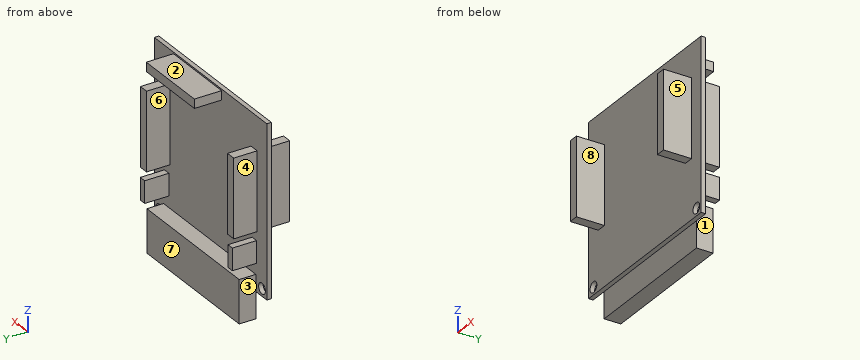
Autodesk Inventor part; units mm, degrees
ref_plane "YZ Plane" through (0, 0, 0) normal (1, 0, 0) x (0, 1, 0)
ref_plane "XZ Plane" through (0, 0, 0) normal (0, 1, 0) x (-1, 0, 0)
ref_plane "XY Plane" through (0, 0, 0) normal (0, 0, 1) x (1, 0, 0)
sketch "Base Board" plane through (0, 0, 0) normal (0, 1, 0) x (-1, 0, 0)
  line L0 (-28.8413, 27.4927) -> (29.6587, 27.4927)
  line L1 (29.6587, 27.4927) -> (29.6587, -28.8073)
  line L2 (29.6587, -28.8073) -> (-28.8413, -28.8073)
  line L3 (-28.8413, -28.8073) -> (-28.8413, 27.4927)
  circle A0 centre (27.1587, -26.3073) radius 1.755
  circle A1 centre (-26.3413, -26.3073) radius 1.755
  line L4 (-23.8413, 16.4927) -> (-20.6413, 16.4927)
  line L5 (-20.6413, 16.4927) -> (-20.6413, -9.3073)
  line L6 (-20.6413, -9.3073) -> (-23.8413, -9.3073)
  line L7 (-23.8413, -9.3073) -> (-23.8413, 16.4927)
  line L8 (24.6587, 16.4927) -> (21.4587, 16.4927)
  line L9 (21.4587, 16.4927) -> (21.4587, -9.3073)
  line L10 (21.4587, -9.3073) -> (24.6587, -9.3073)
  line L11 (24.6587, -9.3073) -> (24.6587, 16.4927)
  point P0 (0, 0)
  dimension "d0" = 58.5
  dimension "d1" = 56.3
  dimension "d2" = 3.51
  dimension "d3" = 2.5
  dimension "d4" = 2.5
  dimension "d5" = 3.51
  dimension "d6" = 2.5
  dimension "d7" = 2.5
  dimension "d19" = 3.2
  dimension "d20" = 25.8
  dimension "d23" = 11
  dimension "d24" = 5
  dimension "d25" = 11
  dimension "d26" = 5
extrude "Base Board Extrusion" add sketch "Base Board" along normal blind 1.5 contours L0 L1 L2 L3 | L4 L5 L6 L7 | L11 L10 L9 L8
sketch "Sketch2" plane through (0, 1.5, 0) normal (0, 1, 0) x (1, 0, 0)
  line L0 (-23.9587, 28.2917) -> (24.0413, 28.2917)
  line L1 (24.0413, 28.2917) -> (24.0413, 23.2917)
  line L2 (24.0413, 23.2917) -> (-23.9587, 23.2917)
  line L3 (-23.9587, 23.2917) -> (-23.9587, 28.2917)
  line L4 (-29.6587, 28.8073) -> (-29.6587, -27.4927)
  point P0 (0, 0)
  dimension "d10" = 48
  dimension "d11" = 5
  dimension "d12" = 5.7
extrude "RightAngleconnectorsBase" add sketch "Sketch2" along normal blind 5.5
sketch "Sketch4" plane through (24.0413, 1.5, -28.2917) normal (0, 0, -1) x (-1, 0, 0)
  line L0 (48, 5.5) -> (0, 5.5)
  line L1 (48, 0) -> (48, 5.5)
  line L2 (0, 5.5) -> (48, 5.5)
  line L3 (48, 5.5) -> (48, 0)
  line L4 (48, 0) -> (0, 0)
  line L5 (0, 0) -> (0, 5.5)
  point P0 (24.0413, -1.5)
extrude "RightAnglePins" add sketch "Sketch4" along normal blind 9.2
extrude "Main IO" add sketch "Base Board" along normal mid plane 18.5 contours L4 L5 L6 L7 | L11 L10 L9 L8
sketch "Sketch6" plane through (0, 1.5, 0) normal (0, 1, 0) x (1, 0, 0)
  line L0 (18.8413, -26.9927) -> (-6.1587, -26.9927)
  line L1 (-6.1587, -26.9927) -> (-6.1587, -23.9927)
  line L2 (-6.1587, -23.9927) -> (18.8413, -23.9927)
  line L3 (18.8413, -23.9927) -> (18.8413, -26.9927)
  line L4 (28.8413, -27.4927) -> (28.8413, 28.8073)
  line L5 (-29.6587, -27.4927) -> (28.8413, -27.4927)
  point P0 (0, 0)
  dimension "d29" = 25
  dimension "d30" = 3
  dimension "d31" = 10
  dimension "d32" = 0.5
extrude "Emulator Pins" add sketch "Sketch6" along normal blind 9
sketch "Sketch7" plane through (0, 1.5, 0) normal (0, 1, 0) x (1, 0, 0)
  line L0 (23.5413, 12.3073) -> (21.2413, 12.3073)
  line L1 (21.2413, 12.3073) -> (21.2413, 19.5573)
  line L2 (21.2413, 19.5573) -> (23.5413, 19.5573)
  line L3 (23.5413, 19.5573) -> (23.5413, 12.3073)
  line L4 (28.8413, -27.4927) -> (28.8413, 28.8073)
  line L5 (23.8413, 9.3073) -> (20.6413, 9.3073)
  line L6 (-29.6587, -27.4927) -> (28.8413, -27.4927)
  line L7 (-24.3587, 12.3073) -> (-22.0587, 12.3073)
  line L8 (-22.0587, 12.3073) -> (-22.0587, 19.5573)
  line L9 (-22.0587, 19.5573) -> (-24.3587, 19.5573)
  line L10 (-24.3587, 19.5573) -> (-24.3587, 12.3073)
  point P0 (0, 0)
  dimension "d35" = 2.3
  dimension "d36" = 7.25
  dimension "d37" = 5.3
  dimension "d38" = 3
extrude "Power Pins" add sketch "Sketch7" along normal blind 8
properties part number "MSP432CoreModule"
Here's how the part is built. I have some questions about the finished solid (model axes, mm). Face numbers are marked on the shaded views. A direction names the side the tool comes from. Round coordinates to 2 decimals unless told otherwise and drop trailing zeros. Write each loop counter-clockwise with the first axis right and the second up, starting at its lowest first coordinate (ties: lowest second). Pieces come first, ordered by that corner, then holes.
Q1. If we section it at D-D on z = 8: Write out the boundary of the cut face in (x, y).
Q2. Will these pins go through, and if not, where does the flat tip stop? P1, Ø5.5, axis at x = 26.34, z = -26.31, coming from the -Y side; P2, Ø6, axis at y = 5, z = 1, coming from the +X side; P3, Ø7, axis at x = 7, z = -34.5, coming from the -Y side.
Q3. If we mould it in two halves opening along X, with no side actions, what happens to the marked faces 5, 6, 7 and 8? For each: +X half, -X half, draft (parallel to the pull), parting line (faces both ways), or undercut.
Q4. If we section it at C-C on x = 0.5: Write out the boundary of the cut face in (y, z).
Q5. If we section it at A-A on y = -6: Write out the boundary of the cut face in (x, z).
Q6. Which directions (+Z, -Z, +X, -X, +Y, -Y) give clear straight access to the entire face, cutting with the end or side of a thin tool? Please do the marked faces 1, 2, 3 and 4.
Q7. If we section it at B-B on y = 4.5: Write out the boundary of the cut face in (x, z), plus the area to 3 significant figures.
Q8. Please list where these lines run through material, in increasing order: probe 1 along X at (y, z) = (2.25, -19); probe 2 along X at (y, z) = (6.75, 1); probe 3 along Y at (x, z) = (22.5, -26.5).
Answer below:
1. outline: (-29.66, 0) - (-24.66, 0) - (-24.66, -9.25) - (-21.46, -9.25) - (-21.46, 0) - (20.64, 0) - (20.64, -9.25) - (23.84, -9.25) - (23.84, 0) - (28.84, 0) - (28.84, 1.5) - (23.84, 1.5) - (23.84, 9.25) - (20.64, 9.25) - (20.64, 1.5) - (-21.46, 1.5) - (-21.46, 9.25) - (-24.66, 9.25) - (-24.66, 1.5) - (-29.66, 1.5) - close
2. P1: stops at y = 0
2. P2: stops at x = 23.84
2. P3: stops at y = 1.5
3. face 5: +X half
3. face 6: undercut
3. face 7: draft
3. face 8: undercut
4. outline: (0, -28.81) - (1.5, -28.81) - (1.5, -37.49) - (7, -37.49) - (7, -23.29) - (1.5, -23.29) - (1.5, 23.99) - (10.5, 23.99) - (10.5, 26.99) - (1.5, 26.99) - (1.5, 27.49) - (0, 27.49) - close
5. outline: (-24.66, -9.31) - (-21.46, -9.31) - (-21.46, 16.49) - (-24.66, 16.49) - close; (20.64, -9.31) - (23.84, -9.31) - (23.84, 16.49) - (20.64, 16.49) - close
6. face 1: +Z, -Z, +X, +Y
6. face 2: +Z, +X, -X, +Y
6. face 3: -Z, -X, +Y
6. face 4: +Z, -Z, -X, +Y
7. outline: (-24.66, -9.31) - (-21.46, -9.31) - (-21.46, 16.49) - (-24.66, 16.49) - close; (-24.36, -19.56) - (-22.06, -19.56) - (-22.06, -12.31) - (-24.36, -12.31) - close; (-23.96, -37.49) - (24.04, -37.49) - (24.04, -23.29) - (-23.96, -23.29) - close; (-6.16, 23.99) - (18.84, 23.99) - (18.84, 26.99) - (-6.16, 26.99) - close; (20.64, -9.31) - (23.84, -9.31) - (23.84, 16.49) - (20.64, 16.49) - close; (21.24, -19.56) - (23.54, -19.56) - (23.54, -12.31) - (21.24, -12.31) - close
7. area: 955 mm2
8. probe 1: x = -24.36 to -22.06, 21.24 to 23.54
8. probe 2: x = -24.66 to -21.46, 20.64 to 23.84
8. probe 3: y = 0 to 7
